Could you check a few things on this model? Use its own coordinates, in mm. A direction names the side the tool comes from. Coordinates: 2 decimals unless noted, no trailing zeros. Order: outer loops, then holes, each group sorted by start corner. A loop starts at its lowest first (then second) coordinate and runs counter-clockwise, first axis right, second up.
```python
from build123d import *

# Parameters (mm, degrees)
F1_DEPTH = 1.5
F3_DEPTH = 1.5
F4_W     = 15.3044191209
F4_H     = 0.5
F5_DEPTH = 12.5
F6_W     = 1.5
F6_H     = 5.51
F7_DEPTH = 2.75


with BuildPart() as f1:
    # F0 (on Top) → F1 (new body)
    with BuildSketch(Plane.XY):
        with BuildLine():
            Line((-31.5180477679, -0.6126557182), (-34.8380477679, -0.6126557182))
            Line((-34.8380477679, -0.6126557182), (-34.8380477679, -9.7026557182))
            Line((-34.8380477679, -9.7026557182), (-29.3529247474, -9.7026557182))
            ThreePointArc((-29.3529247474, -9.7026557182), (-28.0890022814, -10.1526557182), (-26.8250798155, -9.7026557182))
            Line((-26.8250798155, -9.7026557182), (-13.3669702339, -9.7026557182))
            ThreePointArc((-13.3669702339, -9.7026557182), (-12.1030477679, -10.1526557182), (-10.8391253019, -9.7026557182))
            Line((-10.8391253019, -9.7026557182), (2.8830297661, -9.7026557182))
            ThreePointArc((2.8830297661, -9.7026557182), (4.1469522321, -10.1526557182), (5.4108746981, -9.7026557182))
            Line((5.4108746981, -9.7026557182), (19.1330297661, -9.7026557182))
            ThreePointArc((19.1330297661, -9.7026557182), (20.3969522321, -10.1526557182), (21.6608746981, -9.7026557182))
            Line((21.6608746981, -9.7026557182), (24.4319522321, -9.7026557182))
            Line((24.4319522321, -9.7026557182), (24.4319522321, -9.1846820578))
            ThreePointArc((24.4319522321, -9.1846820578), (25.6169859572, -7.3449714109), (24.4319522321, -5.5052607641))
            Line((24.4319522321, -5.5052607641), (24.4319522321, -5.3526557182))
            Line((24.4319522321, -5.3526557182), (32.2019522321, -5.3526557182))
            Line((32.2019522321, -5.3526557182), (32.2019522321, -1.0226557182))
            Line((32.2019522321, -1.0226557182), (24.4319522321, -1.0226557182))
            Line((24.4319522321, -1.0226557182), (24.4319522321, -0.6126557182))
            Line((24.4319522321, -0.6126557182), (23.3219522321, -0.6126557182))
            Line((23.3219522321, -0.6126557182), (21.0319522321, -3.5426557182))
            Line((21.0319522321, -3.5426557182), (22.5319522321, -3.5426557182))
            Line((22.5319522321, -3.5426557182), (22.5319522321, -6.4726557182))
            Line((22.5319522321, -6.4726557182), (18.2619522321, -6.4726557182))
            Line((18.2619522321, -6.4726557182), (16.9619522321, -4.9226557182))
            Line((16.9619522321, -4.9226557182), (16.9619522321, -2.1626557182))
            ThreePointArc((16.9619522321, -2.1626557182), (15.8199018425, -0.3560228098), (13.6980297661, -0.6126557182))
            Line((13.6980297661, -0.6126557182), (7.0719522321, -0.6126557182))
            Line((7.0719522321, -0.6126557182), (4.7819522321, -3.5426557182))
            Line((4.7819522321, -3.5426557182), (6.2819522321, -3.5426557182))
            Line((6.2819522321, -3.5426557182), (6.2819522321, -6.4726557182))
            Line((6.2819522321, -6.4726557182), (2.0119522321, -6.4726557182))
            Line((2.0119522321, -6.4726557182), (0.7119522321, -4.9226557182))
            Line((0.7119522321, -4.9226557182), (0.7119522321, -2.1626557182))
            ThreePointArc((0.7119522321, -2.1626557182), (-0.4300981575, -0.3560228098), (-2.5519702339, -0.6126557182))
            Line((-2.5519702339, -0.6126557182), (-9.1780477679, -0.6126557182))
            Line((-9.1780477679, -0.6126557182), (-11.4680477679, -3.5426557182))
            Line((-11.4680477679, -3.5426557182), (-9.9680477679, -3.5426557182))
            Line((-9.9680477679, -3.5426557182), (-9.9680477679, -6.4726557182))
            Line((-9.9680477679, -6.4726557182), (-14.2380477679, -6.4726557182))
            Line((-14.2380477679, -6.4726557182), (-15.5380477679, -4.9226557182))
            Line((-15.5380477679, -4.9226557182), (-15.5380477679, -2.1626557182))
            ThreePointArc((-15.5380477679, -2.1626557182), (-16.6800981575, -0.3560228098), (-18.8019702339, -0.6126557182))
            Line((-18.8019702339, -0.6126557182), (-25.4880477679, -0.6126557182))
            Line((-25.4880477679, -0.6126557182), (-28.0680477679, -6.5826557182))
            Line((-28.0680477679, -6.5826557182), (-31.5180477679, -6.5826557182))
            Line((-31.5180477679, -6.5826557182), (-31.5180477679, -0.6126557182))
        make_face()
    extrude(amount=F1_DEPTH)

    # F2 (on face) → F3 (join)
    with BuildSketch(Plane.XY.offset(1.5)):
        with BuildLine():
            Line((-31.0880477679, -8.2026557182), (-31.0880477679, -9.7026557182))
            Line((-31.0880477679, -9.7026557182), (-29.3529247474, -9.7026557182))
            ThreePointArc((-29.3529247474, -9.7026557182), (-28.0890022814, -10.1526557182), (-26.8250798155, -9.7026557182))
            Line((-26.8250798155, -9.7026557182), (-13.3669702339, -9.7026557182))
            ThreePointArc((-13.3669702339, -9.7026557182), (-12.1030477679, -10.1526557182), (-10.8391253019, -9.7026557182))
            Line((-10.8391253019, -9.7026557182), (2.8830297661, -9.7026557182))
            ThreePointArc((2.8830297661, -9.7026557182), (4.1469522321, -10.1526557182), (5.4108746981, -9.7026557182))
            Line((5.4108746981, -9.7026557182), (19.1330297661, -9.7026557182))
            ThreePointArc((19.1330297661, -9.7026557182), (20.3969522321, -10.1526557182), (21.6608746981, -9.7026557182))
            Line((21.6608746981, -9.7026557182), (24.4319522321, -9.7026557182))
            Line((24.4319522321, -9.7026557182), (24.4319522321, -9.1846820578))
            Line((24.4319522321, -9.1846820578), (23.5973913223, -9.0155852959))
            Line((23.5973913223, -9.0155852959), (22.8039156646, -8.1339450553))
            Line((22.8039156646, -8.1339450553), (-15.7880477679, -8.1339450553))
            Line((-15.7880477679, -8.1339450553), (-15.7880477679, -4.7026557182))
            Line((-15.7880477679, -4.7026557182), (-17.2880477679, -4.7026557182))
            Line((-17.2880477679, -4.7026557182), (-17.2880477679, -8.2026557182))
            Line((-17.2880477679, -8.2026557182), (-31.0880477679, -8.2026557182))
        make_face()
    extrude(amount=F3_DEPTH)

    # F4 (on face) → F5 (cut, symmetric)
    with BuildSketch(Plane(origin=(0, -8.2026557182, 0), x_dir=(-1, 0, 0), z_dir=(0, 1, 0))):
        with Locations((23.4358382075, 2.75)):
            Rectangle(F4_W, F4_H)
    extrude(amount=F5_DEPTH, both=True, mode=Mode.SUBTRACT)

    # F6 (on face) → F7 (join)
    with BuildSketch(Plane(origin=(0, 0, 0), x_dir=(1, 0, 0), z_dir=(0, 0, -1))):
        with Locations((-34.0880477679, 3.8576557182)):
            Rectangle(F6_W, F6_H)
    extrude(amount=F7_DEPTH)


solid = f1.part
```
Item 1: Which directions (+Z, -Z, +X, -X, +Y, -Y) give clear straight access to the entire face, cutting with the end or side of a thin tool? Please do faces 4 (the face through (22, -3.543, 1)), 5 (the face through (28, -1.023, 1)), 6 (the face through (-10.31, -2.06, 0.74)), 7 (the face through (-20, -9.703, 1)).
Item 2: Suppose I cut it at D-D (x = -21.5). List the corners of the cut face in (y, z) for me, and give its area (3 significant figures).
Item 3: Suppose I cut it at C-C (y = -7.25). List the corners of the cut face in (x, z) for me.
Item 4: I need wall thicknesses on line 1 (Z direction, x = -1.5, y = -5.75); line 2 (Y direction, x = -23.5, z = 2.25); line 3 (X direction, y = -2, z = -0.75). Which ranges of each line are inside material? Lowest first, please.
Item 5: Suppose I cut it at B-B (z = -1.6). List the corners of the cut face in (x, y) for me.
Item 6: Thinking about a two-plate mould opening in Y: for faces 1 (the face through (-11, -3.543, 1)), 2 (the face through (10, -0.613, 1)), 3 (the face through (0.712, -4, 1)), which applies, +Y half, -Y half, draft (parallel to the pull), parting line (faces both ways), or undercut?
Item 7: For pin 1 Ø1.6 at (x, z) = (-22, 0.5) entering from +Y; pin 2 Ø3 at (x, z) = (-17, 2) entering from -Y; pin 3 Ø2 at (x, y) = (-5.5, -4) entering from -Z, each with a flat end and sliding along its axis, tell me the tip position at first contact or that it passes through.
Item 8: Suppose I cut it at A-A (x = -8.5). List the corners of the cut face in (y, z) for me.
Geometry results:
1. face 4: +Z, -Z
1. face 5: +Z, -Z, +X, +Y
1. face 6: +Z, -Z, +Y
1. face 7: +Z, -Z, -Y
2. outline: (-9.7, 0) - (-0.61, 0) - (-0.61, 1.5) - (-8.2, 1.5) - (-8.2, 2.5) - (-9.7, 2.5) - close
2. area: 15.1 mm2
3. outline: (-34.84, 0) - (25.61, 0) - (25.61, 1.5) - (-15.79, 1.5) - (-15.79, 2.5) - (-17.29, 2.5) - (-17.29, 1.5) - (-34.84, 1.5) - close
4. line 1: z = 0 to 1.5
4. line 2: y = -9.7 to -8.2
4. line 3: x = -34.84 to -33.34
5. outline: (-34.84, -6.61) - (-33.34, -6.61) - (-33.34, -1.1) - (-34.84, -1.1) - close
6. face 1: undercut
6. face 2: +Y half
6. face 3: draft
7. pin 1: stops at y = -0.61
7. pin 2: stops at y = -9.7
7. pin 3: stops at z = 0
8. outline: (-9.7, 0) - (-0.61, 0) - (-0.61, 1.5) - (-8.13, 1.5) - (-8.13, 3) - (-9.7, 3) - close
